from build123d import *

# Parameters (mm, degrees)
CROSS_SECTION_SKETCH_R = 15


with BuildPart() as part:
    # Bar Sweep: sweep along a path in Overhead Sketch
    with BuildLine(Plane(origin=(0, 0, 0), x_dir=(1, 0, 0), z_dir=(0, 1, 0))) as bar_sweep_path:
        Line((575.638587088, 200), (705, 200))
        ThreePointArc((705, 200), (726.213203436, 191.213203436), (735, 170))
        Line((735, 170), (735, 0))
        ThreePointArc((735, 0), (644.20543415, -353.870539338), (394.253445956, -620.313807965))
        ThreePointArc((394.253445956, -620.313807965), (371.015343762, -624.131330145), (352.180706456, -609.994877028))
        Line((352.180706456, -609.994877028), (287.5, -497.964607176))
    # Cross Section Sketch → Bar Sweep (sweep)
    with BuildSketch(Plane.ZY.offset(-575.638587088)):
        with Locations((-200, 0)):
            Circle(CROSS_SECTION_SKETCH_R)
    sweep(path=bar_sweep_path.line)


solid = part.part
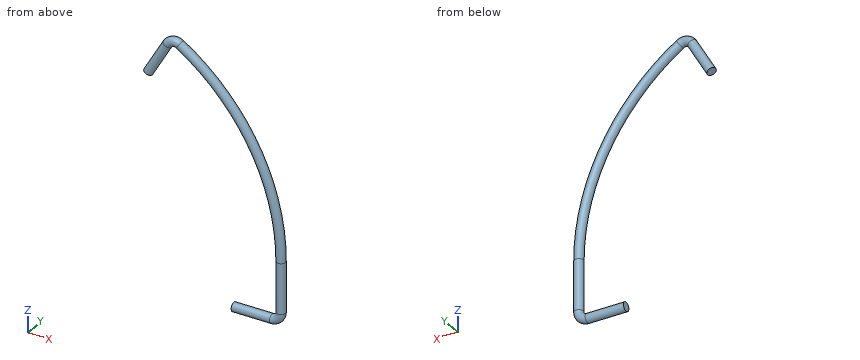
Input: part model. Units: mm. Frame: model coordinates. Coordinates: 2 decimals unless noted, no trailing zeros. Loops run counter-clockwise (first coordinate to the right, second up) from the corner with the lowest first, then second, coordinate; pieces in that order, holes last. Notation, with made-up numbers: (38, 2) -> (60, 2) arc R24 ccw to (60, 24) -> close; hole circle Ø4 at (2.25, 52). An arc over 180 degrees is marked (long way). Write item = value, one per line. Start each with the question number.
Item 1: First-contact query: P1, Ø4, axis at y = -9.5, z = 368, coming from the -X side; P2, Ø2, axis at x = 425.5, y = -1, coming from the +Z side; P3, Ø2, axis at y = -3, z = 123.5, coming from the -X side. Flat tips, straight axial feed; report the tip coordinate or a pass-through.
Item 2: Material intervals for line 1 (X direction, y = -4, z = 511.5); line 2 (Z direction, x = 627.5, y = 6); line 3 (X direction, y = 0, z = -157), sorted ascending.
Item 3: Cut plane A-A, the plane y = 0. Return loops of the section in (x, z).
Item 4: Cut plane B-B, the plane z = -78.5. Return loops of the section in (x, y), plus the area to 3 significant figures.
Ans:
q1.P1 = 620.75
q1.P2 = 618.27
q1.P3 = 709.38
q2.line_1 = 278.62 to 312.01, 507.49 to 547.77
q2.line_2 = -213.75 to -186.25, 355.6 to 408.49
q2.line_3 = 720 to 750
q3.outline = (274.51, 505.46) -> (300.49, 490.46) -> (365.17, 602.49) arc R15 cw to (386.21, 607.65) arc R720 cw to (720, 0) -> (720, -170) arc R15 cw to (705, -185) -> (575.64, -185) -> (575.64, -215) -> (705, -215) arc R45 ccw to (750, -170) -> (750, 0) arc R750 ccw to (402.3, 632.97) arc R45 ccw to (339.19, 617.49) -> close
q4.outline = circle Ø30 at (735, 0)
q4.area = 707 mm²
